Model file for the job. Use its own axes, mm. A direction names the side the tool comes from. Give positions to 0.01 mm unless a question says otherwise; leave off trailing zeros. Loops run counter-clockwise (first coordinate to the right, second up) from the corner with the lowest first, then second, coordinate; pieces in that order, holes last. Notation, with made-up numbers: M -15,22.25 L 4,22.25 A19 cw 4,41.25 Z; hole C 23,-6.5 d2. An arc over 180 degrees is marked long. Answer in a Markdown table with one row per item.
```python
from build123d import *

# Parameters (mm, degrees)
F0_W      = 330.2
F0_H      = 304.8
F1_DEPTH  = 3.175
F2_W      = 76.2
F2_H      = 76.2
F3_DEPTH  = 76.2
F4_W      = 25.4
F4_H      = 152.4
F5_DEPTH  = 25.4
F6_W      = 152.4
F6_H      = 12.7
F7_DEPTH  = 76.2
F8_W      = 127
F8_H      = 50.8
F9_DEPTH  = 38.1
F10_W     = 63.5
F10_H     = 19.05
F11_DEPTH = 25.4
F12_W     = 31.75
F12_H     = 15.875
F13_DEPTH = 25.4


with BuildPart() as f1:
    # F0 (on Top) → F1 (new body)
    with BuildSketch(Plane.XY):
        with Locations((165.1, 152.4)):
            Rectangle(F0_W, F0_H)
    extrude(amount=F1_DEPTH)

    # F2 (on face) → F3 (join)
    with BuildSketch(Plane.XY.offset(3.175)):
        with Locations((266.7, 241.3)):
            Rectangle(F2_W, F2_H)
    extrude(amount=F3_DEPTH)

    # F4 (on face) → F5 (join)
    with BuildSketch(Plane.XY.offset(3.175)):
        with Locations((12.7, 228.6)):
            Rectangle(F4_W, F4_H)
    extrude(amount=F5_DEPTH)

    # F6 (on face) → F7 (join)
    with BuildSketch(Plane.XY.offset(3.175)):
        with Locations((76.2, 107.95)):
            Rectangle(F6_W, F6_H)
    extrude(amount=F7_DEPTH)

    # F8 (on face) → F9 (join)
    with BuildSketch(Plane.XY.offset(3.175)):
        with Locations((254, 152.4)):
            Rectangle(F8_W, F8_H)
    extrude(amount=F9_DEPTH)

    # F10 (on face) → F11 (join)
    with BuildSketch(Plane.XY.offset(3.175)):
        with Locations((273.05, 15.875)):
            Rectangle(F10_W, F10_H)
    extrude(amount=F11_DEPTH)

    # F12 (on face) → F13 (join)
    with BuildSketch(Plane.XY.offset(3.175)):
        with Locations((180.975, 11.1125)):
            Rectangle(F12_W, F12_H)
    extrude(amount=F13_DEPTH)


solid = f1.part
```
(1) Saw through at C-C, the plane x = 32. Give the cut face in (y, z) (3 decimals).
Established:
| item | result |
|---|---|
| outline | M 0,0 L 304.8,0 L 304.8,3.175 L 114.3,3.175 L 114.3,79.375 L 101.6,79.375 L 101.6,3.175 L 0,3.175 Z |
(2) Saw through at D-D, the plane z = 75.5. Give the cut face in (x, y).
Established:
| item | result |
|---|---|
| outline | M 0,101.6 L 152.4,101.6 L 152.4,114.3 L 0,114.3 Z; M 228.6,203.2 L 304.8,203.2 L 304.8,279.4 L 228.6,279.4 Z |
(3) Saw through at A-A, the plane z = 35.5. Give the cut face in (x, y).
Established:
| item | result |
|---|---|
| outline | M 0,101.6 L 152.4,101.6 L 152.4,114.3 L 0,114.3 Z; M 190.5,127 L 317.5,127 L 317.5,177.8 L 190.5,177.8 Z; M 228.6,203.2 L 304.8,203.2 L 304.8,279.4 L 228.6,279.4 Z |
(4) Wall check: L1, parallel to Y at x = 299.5, z = 10; L2, parallel to Y at x = 234, z = 36.5; L3, parallel to X at y = 153, z = 20.5. Give the ranges that are in metal, low to high.
Established:
| item | result |
|---|---|
| L1 | y = 6.35 to 25.4, 127 to 177.8, 203.2 to 279.4 |
| L2 | y = 127 to 177.8, 203.2 to 279.4 |
| L3 | x = 0 to 25.4, 190.5 to 317.5 |
(5) Which spindle directions (+Z, -Z, +X, -X, +Y, -Y) get a long thin tool onto all of the face, cutting with end or side? Do faces 4 (the flat face through (13, 230, 28.575)), 5 (the flat face through (181, 11, 28.575)), 6 (the flat face through (266, 279.4, 41)). Say none if no direction does.
Established:
| item | result |
|---|---|
| face 4 | +Z, -X, +Y |
| face 5 | +Z, +X, -X, -Y |
| face 6 | +Z, +X, +Y |
(6) Saw through at B-B, the plane z = 12.5. Give the cut face in (x, y) (3 decimals), and give its area (3 significant figures).
Established:
| item | result |
|---|---|
| outline | M 0,101.6 L 152.4,101.6 L 152.4,114.3 L 0,114.3 Z; M 0,152.4 L 25.4,152.4 L 25.4,304.8 L 0,304.8 Z; M 165.1,3.175 L 196.85,3.175 L 196.85,19.05 L 165.1,19.05 Z; M 190.5,127 L 317.5,127 L 317.5,177.8 L 190.5,177.8 Z; M 228.6,203.2 L 304.8,203.2 L 304.8,279.4 L 228.6,279.4 Z; M 241.3,6.35 L 304.8,6.35 L 304.8,25.4 L 241.3,25.4 Z |
| area | 19,800 mm2 |
(7) Flat gauge pins, fed straight in: P1, Ø8, axis at y = 10, z = 15.5, coming from the +X side; P2, Ø9.5, axis at y = 13.5, z = 11.5, coming from the -X side; P3, Ø5, axis at x = 256.5, z = 38, coming from the +Y side. Where does each tip first touch, or does it go through?
Established:
| item | result |
|---|---|
| P1 | stops at x = 304.8 |
| P2 | stops at x = 165.1 |
| P3 | stops at y = 279.4 |
(8) Mould opens along Y. For faces 1 (the flat face through (196.85, 11, 16)), 2 (the flat face through (273, 6.35, 16)), 3 (the flat face through (253, 127, 22)) say: pulls with the +Y half, pulls with the -Y half, needs draft (parallel to the pull), parting line crosses it, or undercut.
Established:
| item | result |
|---|---|
| face 1 | needs draft |
| face 2 | pulls with the -Y half |
| face 3 | undercut |
